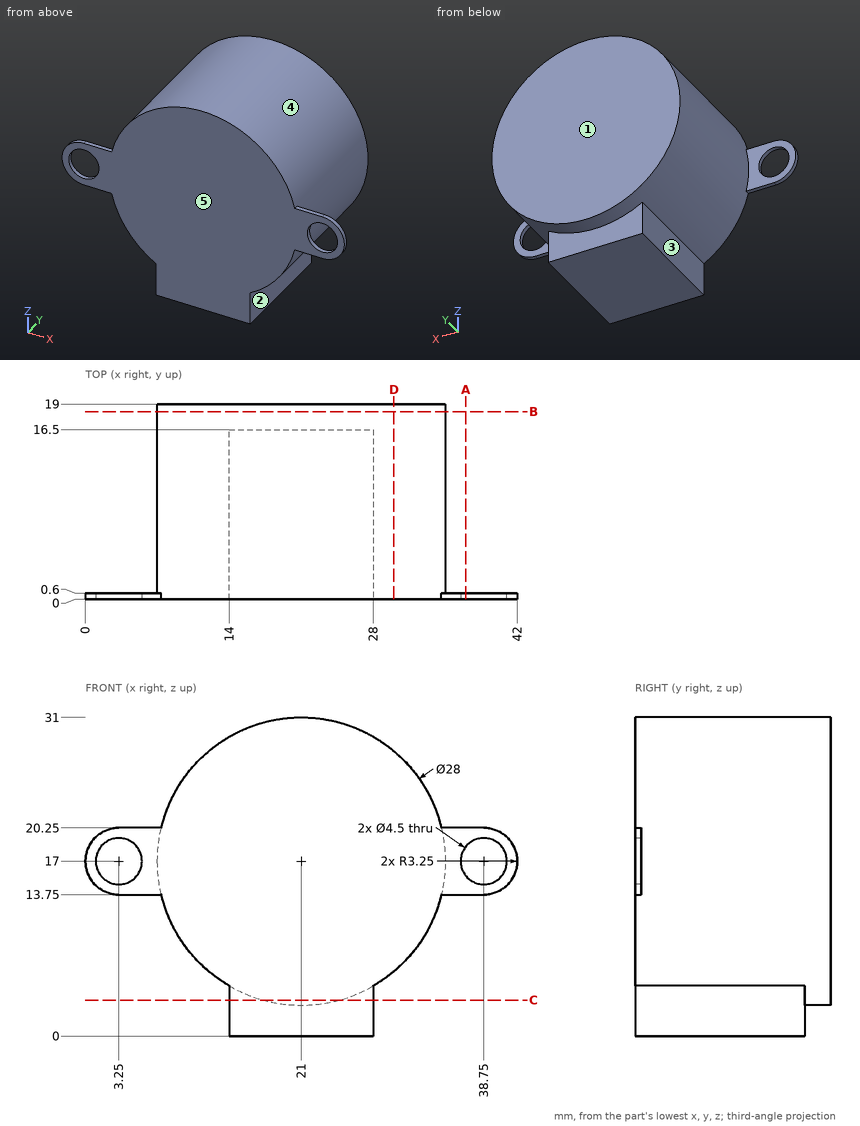
Input: dimensioned drawing with shaded views. Units: mm. Origin: part minimum x, y, z. A direction names the side the tool comes from. Round coordinates to 2 decimals unless told otherwise and drop trailing zeros. Order: outer loops, then holes, each group sorted by start corner. A loop starts at its lowest first (then second) coordinate and runs counter-clockwise, first axis right, second up.
Q1. Pin query (flat end, axial travel): pin 1 (2 mm diameter, centred on x = 37, z = 18, fed in from +Y); pin 2 (2 mm diameter, centred on y = 3.5, z = 13.5, fed in from -X) (3 decimals); pin 3 (0.5 mm diameter, centred on x = 5, y = 0, fed in from +Z); pin 4 (3.5 mm diameter, centred on x = 3.25, z = 17, fed in from +Y). Return the tip coordinate at first contact, or that it passes through.
Result sheet:
pin 1: stops at y = 0.6
pin 2: stops at x = 7.225
pin 3: stops at z = 20.25
pin 4: passes through
Q2. Access query for the marked faces 1, 2, 3, 4 and 5. Directions: +Z, -Z, +X, -X, +Y, -Y. A direction counts if a zero-diameter tool reaches every point of the face in a straight line with its end or side. Return the directions, or none.
Result sheet:
face 1: +Z, -Z, +X, -X, +Y
face 2: -Z, +X, +Y, -Y
face 3: -Z, -X, +Y, -Y
face 4: +Y
face 5: +Z, -Z, +X, -X, -Y
Q3. Section C-C, the plane z = 3.5. Output: boundary loops of the cut face in (x, y), and give its area (3 significant figures).
Result sheet:
outline: (14, 0) - (28, 0) - (28, 16.5) - (24.71, 16.5) - (24.71, 19) - (17.29, 19) - (17.29, 16.5) - (14, 16.5) - close
area: 250 mm2
Q4. Section A-A, the plane x = 37. Output: boundary loops of the cut face in (y, z), and give its area (3 significant figures).
Result sheet:
outline: (0, 13.75) - (0.6, 13.75) - (0.6, 15.59) - (0, 15.59) - close; (0, 18.41) - (0.6, 18.41) - (0.6, 20.25) - (0, 20.25) - close
area: 2.20 mm2
Q5. Section D-D, the plane x = 30. Output: boundary loops of the cut face in (y, z), and give its area (3 significant figures).
Result sheet:
outline: (0, 6.28) - (19, 6.28) - (19, 27.72) - (0, 27.72) - close
area: 408 mm2
Q6. Material intervals for probe 1 along Z at (x, y) = (3.25, 0.4); probe 2 along X at (y, z) = (12.5, 3); probe 3 along X at (y, z) = (10.75, 15), sorted ascending.
Result sheet:
probe 1: z = 13.75 to 14.75, 19.25 to 20.25
probe 2: x = 14 to 28
probe 3: x = 7.14 to 34.86
Q7. Section B-B, the plane y = 18.25. Output: boundary loops of the cut face in (x, z), and give its area (3 significant figures).
Result sheet:
outline: circle Ø28 at (21, 17)
area: 616 mm2
